Design review of the part built by this model. Coordinates are the model's own, in mm. Coordinates: 2 decimals unless noted, no trailing zeros. Write each loop counter-clockwise with the first axis right and the second up, starting at its lowest first coordinate (ties: lowest second). Pieces come first, ordered by that corner, then holes. Notation, with made-up numbers: (84.25, 11.5) -> (132.25, 11.5) arc R13 ccw to (132.25, 19.5) -> close; hole circle Ø5 at (-14, -25.75). An arc over 180 degrees is marked (long way). Write item = value, one per line. Start each with the question number.
```python
from build123d import *

# Parameters (mm, degrees)
SKETCH_W        = 48
SKETCH_H        = 75
PAD_DEPTH       = 1.5
FILLET006_R     = 3
FILLET007_R     = 3
FILLET008_R     = 3
SKETCH010_R     = 1.6
POCKET009_DEPTH = 1.501
SKETCH015_R     = 2.455473
SKETCH015_R_2   = 2.5
POCKET011_DEPTH = 1


with BuildPart() as part:
    # Sketch → Pad (new body)
    with BuildSketch(Plane.XY):
        with Locations((-5, 0)):
            Rectangle(SKETCH_W, SKETCH_H)
    extrude(amount=PAD_DEPTH)

    # Fillet006
    fillet006_edges = [part.edges().sort_by_distance(p)[0] for p in [
        (-29, -37.5, 0.75),
    ]]
    fillet(fillet006_edges, radius=FILLET006_R)

    # Fillet007
    fillet007_edges = [part.edges().sort_by_distance(p)[0] for p in [
        (19, -37.5, 0.75),
        (19, 37.5, 0.75),
    ]]
    fillet(fillet007_edges, radius=FILLET007_R)

    # Fillet008
    fillet008_edges = [part.edges().sort_by_distance(p)[0] for p in [
        (-29, 37.5, 0.75),
    ]]
    fillet(fillet008_edges, radius=FILLET008_R)

    # Sketch010 → Pocket009 (cut, through all)
    with BuildSketch(Plane(origin=(0, 0, 0), x_dir=(1, 0, 0), z_dir=(0, 0, -1))):
        with Locations((-8.375, 33.3)):
            Circle(SKETCH010_R)
        with Locations((8.375, 33.3)):
            Circle(SKETCH010_R)
    extrude(amount=-POCKET009_DEPTH, mode=Mode.SUBTRACT)

    # Sketch015 → Pocket011 (cut)
    with BuildSketch(Plane(origin=(0, 0, 0), x_dir=(1, 0, 0), z_dir=(0, 0, -1))):
        with Locations((-8.375, 33.3)):
            Circle(SKETCH015_R)
        with Locations((8.375, 33.3)):
            Circle(SKETCH015_R_2)
    extrude(amount=-POCKET011_DEPTH, mode=Mode.SUBTRACT)


solid = part.part
```
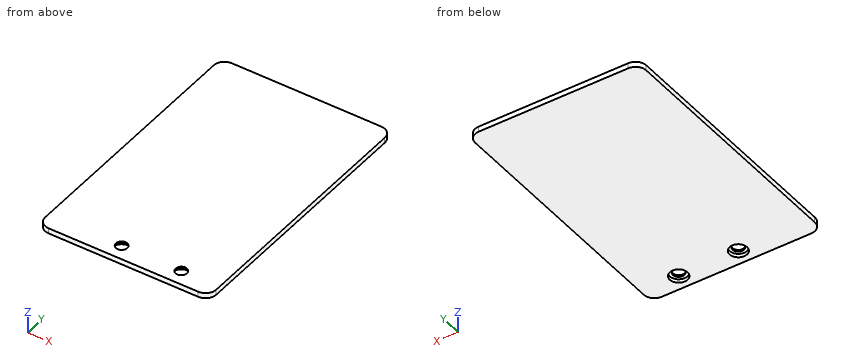
(1) Take a section at A-A, the plane y = -33.3. State the section outline as (x, z) points (3 decimals).
(2) Take a section at B-B, the plane x = -8. State the section outline as (y, z) points, then the cut area to 3 significant figures.
(3) For pin 1 Ø3.5 at (x, y) = (8.375, -33.3) entering from -Z; pin 2 Ø1.9 at (x, y) = (-8.375, -33.3) entering from -Z, all flat-tipped, find the tip position at first contact; note any pin that passes through.
(4) For line 1 (X direction, y = -33.3, z = 0.4) (3 decimals); line 2 (Y direction, x = -8.5, z = 0.15); line 3 (X direction, y = -34, z = 0.85) (3 decimals), list the stretches that pass through material, from the lowest coordinate up.
Report:
q1.outline = (-29, 0) -> (-10.83, 0) -> (-10.83, 1) -> (-9.975, 1) -> (-9.975, 1.5) -> (-29, 1.5) -> close; (-6.775, 1) -> (-5.92, 1) -> (-5.92, 0) -> (5.875, 0) -> (5.875, 1) -> (6.775, 1) -> (6.775, 1.5) -> (-6.775, 1.5) -> close; (9.975, 1) -> (10.875, 1) -> (10.875, 0) -> (19, 0) -> (19, 1.5) -> (9.975, 1.5) -> close
q2.outline = (-37.5, 0) -> (-35.73, 0) -> (-35.73, 1) -> (-34.86, 1) -> (-34.86, 1.5) -> (-37.5, 1.5) -> close; (-31.74, 1) -> (-30.87, 1) -> (-30.87, 0) -> (37.5, 0) -> (37.5, 1.5) -> (-31.74, 1.5) -> close
q2.area = 106 mm2
q3.pin_1 = 1
q3.pin_2 = through
q4.line_1 = -29 to -10.83, -5.92 to 5.875, 10.875 to 19
q4.line_2 = -37.5 to -35.75, -30.85 to 37.5
q4.line_3 = -29 to -10.729, -6.021 to 5.975, 10.775 to 19
